The model under review builds one solid part; all positions refer to its coordinate system, in mm. Coordinates: 2 decimals unless noted, no trailing zeros. Loops run counter-clockwise (first coordinate to the right, second up) from the corner with the lowest first, then second, coordinate; pieces in that order, holes last. Notation, with made-up numbers: M 71,10 L 98,10 A12 cw 98,28 Z; hole C 54,51.25 d2. An arc over 180 degrees is marked long. Use one line per item in the form item = value.
```python
from build123d import *

# Parameters (mm, degrees)
SKETCH_1_W      = 144
SKETCH_1_H      = 66
SKETCH_1_R      = 1.8
SKETCH_1_R_2    = 1.7
EXTRUDE_1_DEPTH = 2.5
FILLET_1_R      = 3.4


with BuildPart() as part:
    # 草图1 → 凸台-拉伸1 (new body)
    with BuildSketch(Plane(origin=(0, 0, 0), x_dir=(1, 0, 0), z_dir=(0, 1, 0))):
        Rectangle(SKETCH_1_W, SKETCH_1_H)
        with Locations(Location((-67, 29, 0), (0, 0, 270))):
            Circle(SKETCH_1_R, mode=Mode.SUBTRACT)
        with Locations(Location((67, 29, 0), (0, 0, 270))):
            Circle(SKETCH_1_R, mode=Mode.SUBTRACT)
        with Locations(Location((-67, -29, 0), (0, 0, 270))):
            Circle(SKETCH_1_R, mode=Mode.SUBTRACT)
        with Locations(Location((67, -29, 0), (0, 0, 270))):
            Circle(SKETCH_1_R, mode=Mode.SUBTRACT)
        with Locations(Location((-67, 0, 0), (0, 0, 270))):
            Circle(SKETCH_1_R_2, mode=Mode.SUBTRACT)
        with Locations(Location((-67, 10.5, 0), (0, 0, 270))):
            Circle(SKETCH_1_R_2, mode=Mode.SUBTRACT)
        with Locations(Location((-67, -10.5, 0), (0, 0, 270))):
            Circle(SKETCH_1_R_2, mode=Mode.SUBTRACT)
        with Locations(Location((67, 0, 0), (0, 0, 270))):
            Circle(SKETCH_1_R_2, mode=Mode.SUBTRACT)
        with Locations(Location((67, 10.5, 0), (0, 0, 270))):
            Circle(SKETCH_1_R_2, mode=Mode.SUBTRACT)
        with Locations(Location((67, -10.5, 0), (0, 0, 270))):
            Circle(SKETCH_1_R_2, mode=Mode.SUBTRACT)
    extrude(amount=EXTRUDE_1_DEPTH)

    # 圆角1
    fillet_1_edges = [part.edges().sort_by_distance(p)[0] for p in [
        (72, 1.25, 33),
        (-72, 1.25, 33),
        (-72, 1.25, -33),
        (72, 1.25, -33),
    ]]
    fillet(fillet_1_edges, radius=FILLET_1_R)


solid = part.part
```
1. Add section B-B (z = -10.5). State the section outline as (x, y) points, then the cut area to 3 significant figures.
Response values:
outline = M -72,0 L -68.7,0 L -68.7,2.5 L -72,2.5 Z; M -65.3,0 L 65.3,0 L 65.3,2.5 L -65.3,2.5 Z; M 68.7,0 L 72,0 L 72,2.5 L 68.7,2.5 Z
area = 343 mm^2
2. The part is to be moulded in two halves that separate along Z. For faces 1 (the face through (65.5, 1.2, -9.7)), 2 (the face through (72, 1, 0)), 3 (the face through (70.98, 1.27, -32.03)), say which applies: pulls with the +Z half, pulls with the -Z half, needs draft (parallel to the pull), parting line crosses it, or undercut.
Response values:
face_1 = undercut
face_2 = needs draft
face_3 = pulls with the -Z half
3. Add section A-A (x = 67). State the section outline as (y, z) points, then the cut area to 4 significant figures.
Response values:
outline = M 0,-33 L 2.5,-33 L 2.5,-30.8 L 0,-30.8 Z; M 0,-27.2 L 2.5,-27.2 L 2.5,-12.2 L 0,-12.2 Z; M 0,-8.8 L 2.5,-8.8 L 2.5,-1.7 L 0,-1.7 Z; M 0,1.7 L 2.5,1.7 L 2.5,8.8 L 0,8.8 Z; M 0,12.2 L 2.5,12.2 L 2.5,27.2 L 0,27.2 Z; M 0,30.8 L 2.5,30.8 L 2.5,33 L 0,33 Z
area = 121.5 mm^2
4. Wall thickness on line 1 along X through (y, z) = (1.2, -29); line 2 along Z through (x, y) = (67, 1.55); line 3 along X through (y, z) = (1.1, 29.5): over which ranges is each line inside the solid? List them lowest first. Write a range as from..to.
Response values:
line_1 = -72..-68.8, -65.2..65.2, 68.8..72
line_2 = -33..-30.8, -27.2..-12.2, -8.8..-1.7, 1.7..8.8, 12.2..27.2, 30.8..33
line_3 = -72..-68.73, -65.27..65.27, 68.73..72
